from build123d import *

# Parameters (mm, degrees)
SKETCH_2_R          = 6.05
SKETCH_2_R_2        = 2.05
EXTRUDE_1_DEPTH     = 5
EXTRUDE_1_2_DEPTH   = 5
EXTRUDE_1_3_DEPTH   = 5
EXTRUDE_1_4_DEPTH   = 5
SKETCH_6_R          = 2.05
EXTRUDE_1_5_DEPTH   = 5
SKETCH_7_W          = 14.3
SKETCH_7_H          = 45.6
SKETCH_7_W_2        = 9.5
SKETCH_7_H_2        = 8.2
SKETCH_7_W_3        = 8
SKETCH_7_H_3        = 11
SKETCH_7_W_4        = 17
CUT_EXTRUDE_1_DEPTH = 5


with BuildPart() as part:
    # 草图2 → Extrude 1 (new body)
    with BuildSketch(Plane(origin=(0, 0, 0), x_dir=(-1, 0, 0), z_dir=(0, -1, 0))):
        with Locations((-103.2, -9.35)):
            Circle(SKETCH_2_R)
        with Locations((-103.2, -9.35)):
            Circle(SKETCH_2_R_2, mode=Mode.SUBTRACT)
    extrude(amount=EXTRUDE_1_DEPTH)



with BuildPart() as body_2:
    # 草图2 → Extrude 1 2 (new body)
    with BuildSketch(Plane(origin=(0, 0, 0), x_dir=(-1, 0, 0), z_dir=(0, -1, 0))):
        with Locations((-59.2, -9.35)):
            Circle(SKETCH_2_R)
        with Locations((-59.2, -9.35)):
            Circle(SKETCH_2_R_2, mode=Mode.SUBTRACT)
    extrude(amount=EXTRUDE_1_2_DEPTH)


with BuildPart() as body_3:
    # 草图2 → Extrude 1 3 (new body)
    with BuildSketch(Plane(origin=(0, 0, 0), x_dir=(-1, 0, 0), z_dir=(0, -1, 0))):
        with Locations((-59.2, -64.25)):
            Circle(SKETCH_2_R)
        with Locations((-59.2, -64.25)):
            Circle(SKETCH_2_R_2, mode=Mode.SUBTRACT)
    extrude(amount=EXTRUDE_1_3_DEPTH)


with BuildPart() as body_4:
    # 草图2 → Extrude 1 4 (new body)
    with BuildSketch(Plane(origin=(0, 0, 0), x_dir=(-1, 0, 0), z_dir=(0, -1, 0))):
        with Locations((-103.2, -64.25)):
            Circle(SKETCH_2_R)
        with Locations((-103.2, -64.25)):
            Circle(SKETCH_2_R_2, mode=Mode.SUBTRACT)
    extrude(amount=EXTRUDE_1_4_DEPTH)


with BuildPart() as part_1:
    add(part.part)

    add(body_2.part)  # Extrude 1 5 merges body 2

    add(body_3.part)  # Extrude 1 5 merges body 3

    add(body_4.part)  # Extrude 1 5 merges body 4
    # 草图6 → Extrude 1 5 (add)
    with BuildSketch(Plane(origin=(0, 0, 0), x_dir=(1, 0, 0), z_dir=(0, 1, 0))):
        with BuildLine():
            Line((107.197188412, -4.808526143), (124.864153797, -20.358145394))
            ThreePointArc((124.864153797, -20.358145394), (126.367399875, -22.390742927), (126.9, -24.862086409))
            Line((126.9, -24.862086409), (126.9, -68.95))
            ThreePointArc((126.9, -68.95), (125.142640687, -73.192640687), (120.9, -74.95))
            Line((120.9, -74.95), (109.046152581, -74.95))
            ThreePointArc((109.046152581, -74.95), (105.311182702, -73.645742753), (103.2, -70.3))
            Line((103.2, -70.3), (48.2, -70.3))
            ThreePointArc((48.2, -70.3), (43.957359313, -68.542640687), (42.2, -64.3))
            Line((42.2, -64.3), (42.2, -9.35))
            ThreePointArc((42.2, -9.35), (43.972003974, -5.072003974), (48.25, -3.3))
            Line((48.25, -3.3), (59.2, -3.3))
            Line((59.2, -3.3), (103.2, -3.3))
            ThreePointArc((103.2, -3.3), (105.336186224, -3.689681244), (107.197188412, -4.808526143))
        make_face()
        with Locations(Location((103.2, -9.35, 0), (0, 0, 270))):
            Circle(SKETCH_6_R, mode=Mode.SUBTRACT)
        with Locations(Location((103.2, -64.25, 0), (0, 0, 270))):
            Circle(SKETCH_6_R, mode=Mode.SUBTRACT)
        with Locations(Location((59.2, -64.25, 0), (0, 0, 270))):
            Circle(SKETCH_6_R, mode=Mode.SUBTRACT)
        with Locations(Location((59.2, -9.35, 0), (0, 0, 90))):
            Circle(SKETCH_6_R, mode=Mode.SUBTRACT)
    extrude(amount=-EXTRUDE_1_5_DEPTH)

    # 草图7 → 切除-拉伸1 (cut)
    with BuildSketch(Plane(origin=(0, -5, 3), x_dir=(1, 0, 0), z_dir=(0, -1, 0))):
        with Locations((115.75, 44.5)):
            Rectangle(SKETCH_7_W, SKETCH_7_H)
        with Locations((102.95, 19.45)):
            Rectangle(SKETCH_7_W_2, SKETCH_7_H_2)
        with Locations((93.9, 31.05)):
            Rectangle(SKETCH_7_W_3, SKETCH_7_H_3)
        with Locations((83.7, 19.45)):
            Rectangle(SKETCH_7_W_4, SKETCH_7_H_2)
        Polygon((72.4, 24.35), (72.4, 15.35), (66.4, 15.35), (66.4, 10.15), (47.4, 10.15), (47.4, 33.65), (50.4, 33.65), (50.4, 54.65), (85.4, 54.65), (85.4, 48.65), (80.4, 48.65), (80.4, 33.65), (66.4, 33.65), (66.4, 24.35), align=None)
    extrude(amount=-CUT_EXTRUDE_1_DEPTH, mode=Mode.SUBTRACT)


solid = part_1.part
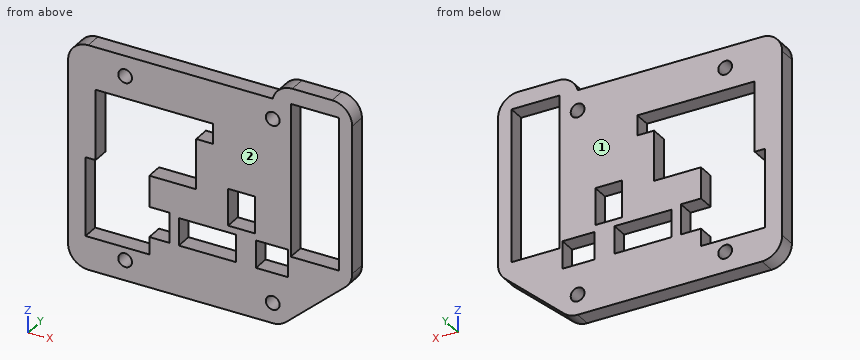
Read the model definition and answer for the solid it produces. Units are mm, in the model's axes. Face numbers are marked on the shaded views. Round coordinates to 2 decimals unless told otherwise and drop trailing zeros. Write each loop counter-clockwise with the first axis right and the second up, starting at its lowest first coordinate (ties: lowest second). Pieces come first, ordered by that corner, then holes. Notation, with made-up numbers: (46.25, 79) - (55.25, 79) arc R21 cw to (55.25, 102) - close; hole circle Ø8 at (48.5, 15). An arc over 180 degrees is marked (long way). One line per question, with ' | ' between items. Start each with the question number.
1. Find the intervals of material crossed by probe 1 along X at (y, z) = (-3.75, 38.5); probe 2 along X at (y, z) = (-3.95, 64.25); probe 3 along Z at (x, y) = (59.5, -3.05), in increasing order. Write a range as [from, to].
2. Section D-D (y = -3.3) is taken. Give the number of separate pieces and of enclosed holes in the cut face, and give its area (3 significant figures).
3. Section A-A (x = 59.2) is taken. Determine the outline of the cut face in (y, z).
4. Each of these flat-tipped pins is pushed along its axis until it touches: pin 1 (6 mm diameter, centred on x = 63.5, z = 15.5, fed in from -Y); pin 2 (2.5 mm diameter, centred on x = 52.5, y = -3, fed in from +Z). Where does it stop, or does it pass through?
5. For a pull along Y with two mould halves and no side action, classify the marked faces 1 and 2 as +Y half, -Y half, draft (parallel to the pull), parting line (faces both ways), or undercut.
6. Section C-C (x = 112.5) is taken. Determine the outline of the cut face in (y, z), and give its area (3 significant figures).
7. Section B-B (z = 17) is taken. Determine the outline of the cut face in (x, y).
Filled in:
1) probe 1: [42.2, 50.4], [80.4, 89.9], [97.9, 108.6], [122.9, 126.9] | probe 2: [42.2, 57.15], [61.25, 101.15], [105.25, 108.6], [122.9, 126.9] | probe 3: [3.3, 7.32], [11.38, 13.15], [57.65, 62.22], [66.28, 70.3]
2) separate pieces: 1 | enclosed holes: 9 | area: 3,380 mm²
3) outline: (-5, 3.3) - (0, 3.3) - (0, 7.3) - (-5, 7.3) - close; (-5, 11.4) - (0, 11.4) - (0, 13.15) - (-5, 13.15) - close; (-5, 57.65) - (0, 57.65) - (0, 62.2) - (-5, 62.2) - close; (-5, 66.3) - (0, 66.3) - (0, 70.3) - (-5, 70.3) - close
4) pin 1: y = -5 | pin 2: z = 70.3
5) face 1: +Y half | face 2: -Y half
6) outline: (-5, 9.48) - (0, 9.48) - (0, 24.7) - (-5, 24.7) - close; (-5, 70.3) - (0, 70.3) - (0, 74.95) - (-5, 74.95) - close | area: 99.4 mm²
7) outline: (42.2, -5) - (47.4, -5) - (47.4, 0) - (42.2, 0) - close; (66.4, -5) - (121.05, -5) - (121.05, 0) - (66.4, 0) - close
